Verification items for the finished model (mm, model axes). Face numbers are marked on the shaded views. A direction names the side the tool comes from. Round coordinates to 2 decimals unless told otherwise and drop trailing zeros. Order: outer loops, then holes, each group sorted by start corner. A loop starts at its lowest first (then second) coordinate and runs counter-clockwise, first axis right, second up. Notation, with made-up numbers: M 23,89.5 L 70,89.5 A27 cw 70,128.5 Z; hole C 85.5,86.25 d1. An arc over 180 degrees is marked long. Use one line per item in the form item = value. Start each with the question number.
Item 1: Release check for a two-part mould opening along Y. For the marked faces 1, 2 and 3 record: +Y half, -Y half, draft (parallel to the pull), parting line (faces both ways), or undercut.
Item 2: Go/stop test with a flat-tipped pin: pin 1 Ø10.5 at (x, z) = (30, 0) entering from +Y. Record where the tip stops, or that it passes through.
Item 3: Thickness scan on probe 1 along X at (y, z) = (2.4, 0); probe 2 along Z at (x, y) = (-30, 1.3); probe 3 along Z at (x, y) = (-30, 27.5). Record the ranges inside material, lowest first. Write a range as [from, to].
Item 4: Cross-section at C-C on z = 0. Enter the section's corners in (x, y), then the cut area to 3 significant figures.
Item 5: Cross-section at B-B on y = 6.5. Enter the section's corners in (x, z).
Item 6: Tool access check on the marked faces 4 and 5. Record the directions out of +Z, -Z, +X, -X, +Y, -Y that give a thin tool (end or side, any length) a straight path to the whole face; none if there is none.
Item 7: Cross-section at A-A on x = 30. Enter the section's corners in (y, z).
Item 8: Cross-section at D-D on x = 13. Enter the section's corners in (y, z), then the cut area to 3 significant figures.
from build123d import *

# Parameters (mm, degrees)
EXTRUDE_1_DEPTH     = 100
SKETCH_2_R          = 4
CUT_EXTRUDE_1_DEPTH = 62.64414003


with BuildPart() as part:
    # 草图1 → 凸台-拉伸1 (new body)
    with BuildSketch(Plane(origin=(-50, 0, 0), x_dir=(0, 0, -1), z_dir=(1, 0, 0))):
        Polygon((20, 0), (-20, 0), (-20, 30), (-16, 30), (-16, 4), (16, 4), (16, 30), (20, 30), align=None)
    extrude(amount=EXTRUDE_1_DEPTH)

    # 草图2 → 切除-拉伸1 (cut, through all)
    with BuildSketch(Plane(origin=(0, 0, 0), x_dir=(1, 0, 0), z_dir=(0, 1, 0))):
        with Locations(Location((-30, 0, 0), (0, 0, 90))):
            Circle(SKETCH_2_R)
        with Locations(Location((0, 0, 0), (0, 0, 90))):
            Circle(SKETCH_2_R)
        with Locations(Location((30, 0, 0), (0, 0, 90))):
            Circle(SKETCH_2_R)
    extrude(amount=CUT_EXTRUDE_1_DEPTH, mode=Mode.SUBTRACT)


solid = part.part
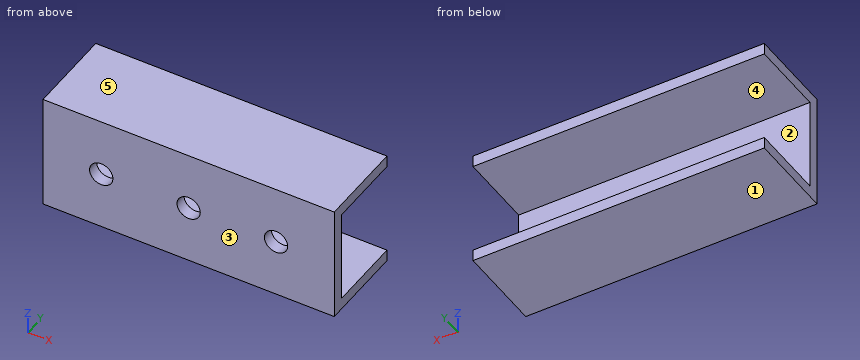
Output values:
q1.face_1 = draft
q1.face_2 = +Y half
q1.face_3 = -Y half
q2.pin_1 = 4
q3.probe_1 = [-50, -34], [-26, -4], [4, 26], [34, 50]
q3.probe_2 = [-20, -4], [4, 20]
q3.probe_3 = [-20, -16], [16, 20]
q4.outline = M -50,0 L -34,0 L -34,4 L -50,4 Z; M -26,0 L -4,0 L -4,4 L -26,4 Z; M 4,0 L 26,0 L 26,4 L 4,4 Z; M 34,0 L 50,0 L 50,4 L 34,4 Z
q4.area = 304 mm2
q5.outline = M -50,-20 L 50,-20 L 50,-16 L -50,-16 Z; M -50,16 L 50,16 L 50,20 L -50,20 Z
q6.face_4 = +X, -X, +Y
q6.face_5 = +Z, +X, -X, +Y, -Y
q7.outline = M 0,-20 L 30,-20 L 30,-16 L 4,-16 L 4,-4 L 0,-4 Z; M 0,4 L 4,4 L 4,16 L 30,16 L 30,20 L 0,20 Z
q8.outline = M 0,-20 L 30,-20 L 30,-16 L 4,-16 L 4,16 L 30,16 L 30,20 L 0,20 Z
q8.area = 368 mm2
